Read the model definition and answer for the solid it produces. Units are mm, in the model's axes. A direction names the side the tool comes from. Coordinates: 2 decimals unless noted, no trailing zeros. Write each loop counter-clockwise with the first axis right and the second up, starting at its lowest first coordinate (ties: lowest second). Pieces come first, ordered by that corner, then holes. Notation, with made-up numbers: M -17.5,64 L -1.5,64 A21 ccw -1.5,73 Z; hole C 65,-27 d10. An arc over 180 degrees is marked long. Write item = value, one per line.
Autodesk Inventor part; units mm, degrees
ref_plane "YZ Plane" through (0, 0, 0) normal (1, 0, 0) x (0, 1, 0)
ref_plane "XZ Plane" through (0, 0, 0) normal (0, 1, 0) x (-1, 0, 0)
ref_plane "XY Plane" through (0, 0, 0) normal (0, 0, 1) x (1, 0, 0)
sketch "Sketch1" plane through (0, 0, 0) normal (0, 0, 1) x (1, 0, 0)
  circle A0 centre (0, 0) radius 4
  circle A1 centre (0, 0) radius 2.26
  dimension "d0" = 8
  dimension "d1" = 4.52
extrude "Extrusion1" add sketch "Sketch1" along normal blind 5.75
sketch "Sketch2" plane through (0, 0, 0) normal (0, 0, -1) x (-1, 0, 0)
  circle A0 centre (0, 0) radius 2.26
  circle A1 centre (6, 0) radius 1
  circle A2 centre (-6, 0) radius 1
  line L0 (8, 4) -> (-8, 4)
  line L1 (-8, 4) -> (-8, -4)
  line L2 (-8, -4) -> (8, -4)
  line L3 (8, -4) -> (8, 4)
  line L4 (8, 4) -> (-8, -4) construction
  line L5 (-8, 4) -> (8, -4) construction
  dimension "d7" = 2
  dimension "d8" = 2
  dimension "d9" = 6
  dimension "d10" = 6
  dimension "d11" = 0
  dimension "d12" = 0
  dimension "d19" = 16
  dimension "d20" = 8
extrude "Extrusion2" add sketch "Sketch2" against normal blind 3
fillet "Fillet1" radius 1 4 edges at (8, 4, 1.5) (8, -4, 1.5) (-8, -4, 1.5) (-8, 4, 1.5)
equation "\"d29\" = 55deg"
equation "\"Sketch3_Pitch\" = 0.8"
equation "\"d47\" = 55deg"
equation "\"Sketch5_Pitch\" = 0.4"
equation "\"d65\" = 55deg"
equation "\"Sketch7_Pitch\" = 0.4"
properties part number "M5Nut_Special"
Item 1: A flat-ended cylindrical pin translates along its axis: pin 1 (3 mm diameter, centred on x = -6, y = 0, fed in from +Z). Find the tip coordinate at first contact, or state that the pin passes through.
Worked answers:
pin_1 = 3
Item 2: For a pull along Y with two mould halves and no side action, classify faces 4 (the face through (-5.2, -0.6, 1.5)), 5 (the face through (0, -4, 1)), 6 (the face through (-8, 0, 1)) as released by +Y, released by -Y, zero draft, split by the parting line, or undercut.
Worked answers:
face_4 = undercut
face_5 = released by -Y
face_6 = zero draft
Item 3: Consider line 1 along Y through (x, z) = (6, 0.7); line 2 along Y through (x, z) = (0, 2.7); line 3 along Z through (x, y) = (-3.5, 2). Determine where each line is inside the solid, lowest interval first. Write a range as from..to.
Worked answers:
line_1 = -4..-1, 1..4
line_2 = -4..-2.26, 2.26..4
line_3 = 0..3
Item 4: Which of the six approach directions +Z, -Z, +X, -X, +Y, -Y give full straight-line access (tool end or side, diameter ignored) to faces 1 (the face through (-4.8, 0.1, 3)), 2 (the face through (8, 0, 1)), 3 (the face through (-0.867, 3.905, 4.356))?
Worked answers:
face_1 = +Z, -X
face_2 = +Z, -Z, +X, +Y, -Y
face_3 = +Z
Item 5: Find section C-C (x = -6). Determine the outline of the cut face in (y, z), and give its area (3 significant figures).
Worked answers:
outline = M -4,0 L -1,0 L -1,3 L -4,3 Z; M 1,0 L 4,0 L 4,3 L 1,3 Z
area = 18.0 mm²
Item 6: Find section B-B (z = 2.35). Determine the outline of the cut face in (x, y), and give its area (3 significant figures).
Worked answers:
outline = M -8,-3 A1 ccw -7,-4 L 7,-4 A1 ccw 8,-3 L 8,3 A1 ccw 7,4 L -7,4 A1 ccw -8,3 Z; hole C -6,0 d2; hole C 0,0 d4.52; hole C 6,0 d2
area = 105 mm²
Item 7: Find section D-D (y = -2). Determine the outline of the cut face in (x, z), and give its area (3 significant figures).
Worked answers:
outline = M -8,0 L -1.05,0 L -1.05,5.75 L -3.46,5.75 L -3.46,3 L -8,3 Z; M 1.05,0 L 8,0 L 8,3 L 3.46,3 L 3.46,5.75 L 1.05,5.75 Z
area = 54.9 mm²
Item 8: Find section A-A (y = 0). Determine the outline of the cut face in (x, z), and give its area (3 significant figures).
Worked answers:
outline = M -8,0 L -7,0 L -7,3 L -8,3 Z; M -5,0 L -2.26,0 L -2.26,5.75 L -4,5.75 L -4,3 L -5,3 Z; M 2.26,0 L 5,0 L 5,3 L 4,3 L 4,5.75 L 2.26,5.75 Z; M 7,0 L 8,0 L 8,3 L 7,3 Z
area = 32.0 mm²
